Can you work these out from the model? Positions are in its coordinate system, mm. Face numbers are marked on the shaded views. A direction names the side the tool comes from. Coordinates: 2 decimals unless noted, no trailing zeros. Order: outer loops, then holes, each group sorted by start corner. A loop starts at its lowest first (then second) coordinate and runs counter-clockwise, first axis right, second up. Notation, with made-up numbers: (-30, -19) -> (12, -19) arc R21 ccw to (12, 14) -> close; hole circle Ø11 at (22.5, -13.5). An arc over 180 degrees is marked (long way). Write item = value, one per line. Start each with the question number.
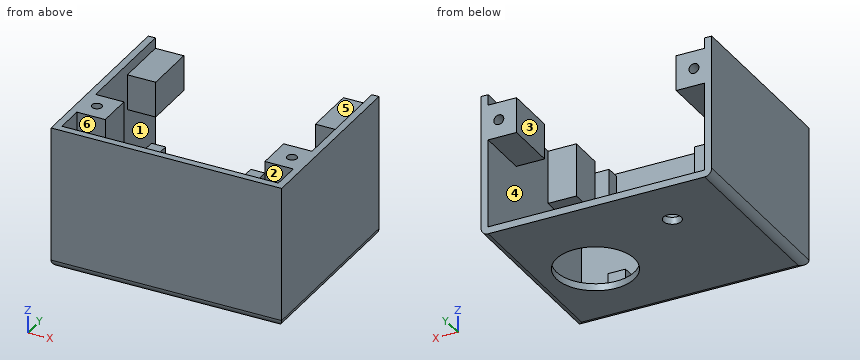
from build123d import *

# Parameters (mm, degrees)
SKETCH1_W           = 65
SKETCH1_H           = 52
BOSS_EXTRUDE1_DEPTH = 40
SHELL1_T            = -2
SKETCH7_W           = 10
SKETCH7_H           = 10
BOSS_EXTRUDE3_DEPTH = 15
SKETCH8_R           = 1.4
CUT_EXTRUDE3_DEPTH  = 10
SKETCH10_W          = 10
SKETCH10_H          = 10
BOSS_EXTRUDE4_DEPTH = 15
SKETCH11_R          = 1.4
CUT_EXTRUDE4_DEPTH  = 10
SKETCH13_R          = 2.5
CUT_EXTRUDE5_DEPTH  = 2
SKETCH16_W          = 10
SKETCH16_H          = 4
BOSS_EXTRUDE5_DEPTH = 13
SKETCH17_W          = 10
SKETCH17_H          = 2
CUT_EXTRUDE6_DEPTH  = 3
SKETCH18_W          = 4
SKETCH18_H          = 4
BOSS_EXTRUDE6_DEPTH = 10
SKETCH20_W          = 4
SKETCH20_H          = 4
BOSS_EXTRUDE7_DEPTH = 10
FILLET1_R           = 2
SKETCH22_W          = 5
SKETCH22_H          = 5
BOSS_EXTRUDE8_DEPTH = 3
SKETCH23_W          = 5
SKETCH23_H          = 5
BOSS_EXTRUDE9_DEPTH = 3
SKETCH24_R          = 11
CUT_EXTRUDE7_DEPTH  = 2


with BuildPart() as part:
    # Sketch1 → Boss-Extrude1 (new body)
    with BuildSketch(Plane.XY):
        with Locations((32.5, 26)):
            Rectangle(SKETCH1_W, SKETCH1_H)
    extrude(amount=BOSS_EXTRUDE1_DEPTH)

    # Shell1
    shell1_openings = [part.faces().sort_by_distance(p)[0] for p in [
        (32.5, 26, 40),
        (32.5, 52, 20),
    ]]
    offset(amount=SHELL1_T, openings=shell1_openings, kind=Kind.INTERSECTION)

    # Sketch7 → Boss-Extrude3 (add)
    with BuildSketch(Plane(origin=(0, 52, 0), x_dir=(1, 0, 0), z_dir=(0, 1, 0))):
        with Locations((5, -32)):
            Rectangle(SKETCH7_W, SKETCH7_H)
    boss_extrude3 = extrude(amount=-BOSS_EXTRUDE3_DEPTH)

    # Sketch8 → Cut-Extrude3 (cut)
    with BuildSketch(Plane(origin=(0, 52, 0), x_dir=(1, 0, 0), z_dir=(0, 1, 0))):
        with Locations((5, -32)):
            Circle(SKETCH8_R)
    cut_extrude3 = extrude(amount=-CUT_EXTRUDE3_DEPTH, mode=Mode.SUBTRACT)

    # Mirror3: Boss-Extrude3, Cut-Extrude3 across plane
    add(boss_extrude3.mirror(Plane(origin=(32.5, 0, 0), x_dir=(0, 0, 1), z_dir=(1, 0, 0))))
    add(cut_extrude3.mirror(Plane(origin=(32.5, 0, 0), x_dir=(0, 0, 1), z_dir=(1, 0, 0))), mode=Mode.SUBTRACT)

    # Sketch10 → Boss-Extrude4 (add)
    with BuildSketch(Plane.XY.offset(40)):
        with Locations((5, 15)):
            Rectangle(SKETCH10_W, SKETCH10_H)
    boss_extrude4 = extrude(amount=-BOSS_EXTRUDE4_DEPTH)

    # Sketch11 → Cut-Extrude4 (cut)
    with BuildSketch(Plane.XY.offset(40)):
        with Locations((5, 15)):
            Circle(SKETCH11_R)
    cut_extrude4 = extrude(amount=-CUT_EXTRUDE4_DEPTH, mode=Mode.SUBTRACT)

    # Mirror4: Boss-Extrude4, Cut-Extrude4 across plane
    add(boss_extrude4.mirror(Plane(origin=(32.5, 0, 0), x_dir=(0, 0, 1), z_dir=(1, 0, 0))))
    add(cut_extrude4.mirror(Plane(origin=(32.5, 0, 0), x_dir=(0, 0, 1), z_dir=(1, 0, 0))), mode=Mode.SUBTRACT)

    # Sketch13 → Cut-Extrude5 (cut)
    with BuildSketch(Plane(origin=(0, 0, 0), x_dir=(-1, 0, 0), z_dir=(0, 0, -1))):
        with Locations((-19, 37)):
            Circle(SKETCH13_R)
    extrude(amount=-CUT_EXTRUDE5_DEPTH, mode=Mode.SUBTRACT)

    # Sketch16 → Boss-Extrude5 (add)
    with BuildSketch(Plane.XY.offset(2)):
        with Locations((19, 6)):
            Rectangle(SKETCH16_W, SKETCH16_H)
    extrude(amount=BOSS_EXTRUDE5_DEPTH)

    # Sketch17 → Cut-Extrude6 (cut)
    with BuildSketch(Plane.XY.offset(15)):
        with Locations((19, 7)):
            Rectangle(SKETCH17_W, SKETCH17_H)
    extrude(amount=-CUT_EXTRUDE6_DEPTH, mode=Mode.SUBTRACT)

    # Sketch18 → Boss-Extrude6 (add)
    with BuildSketch(Plane.XY.offset(2)):
        with Locations((33, 46)):
            Rectangle(SKETCH18_W, SKETCH18_H)
    extrude(amount=BOSS_EXTRUDE6_DEPTH)

    # Sketch20 → Boss-Extrude7 (add)
    with BuildSketch(Plane.XY.offset(2)):
        with Locations((5, 46)):
            Rectangle(SKETCH20_W, SKETCH20_H)
    extrude(amount=BOSS_EXTRUDE7_DEPTH)

    # Fillet1
    fillet1_edges = [part.edges().sort_by_distance(p)[0] for p in [
        (65, 26, 0),
        (32.5, 0, 0),
        (0, 26, 0),
    ]]
    fillet(fillet1_edges, radius=FILLET1_R)

    # Sketch22 → Boss-Extrude8 (add)
    with BuildSketch(Plane.XY.offset(2)):
        with Locations((47.5, 37.8)):
            Rectangle(SKETCH22_W, SKETCH22_H)
    extrude(amount=BOSS_EXTRUDE8_DEPTH)

    # Sketch23 → Boss-Extrude9 (add)
    with BuildSketch(Plane.XY.offset(2)):
        with Locations((47.5, 10.2)):
            Rectangle(SKETCH23_W, SKETCH23_H)
    extrude(amount=BOSS_EXTRUDE9_DEPTH)

    # Sketch24 → Cut-Extrude7 (cut)
    with BuildSketch(Plane.XY.offset(2)):
        with Locations((47.5, 24.03)):
            Circle(SKETCH24_R)
    extrude(amount=-CUT_EXTRUDE7_DEPTH, mode=Mode.SUBTRACT)


solid = part.part
(1) If I drill on L1, parallel to Z at x = 60, y = 44.5; L2, parallel to Y at x = 56, z = 35; L3, parallel to X at y = 34, z = 19.5, over which ranges is the centre line in solid material (lowest first)? Write a range as from..to.
(2) For the marked faces 1, 2 and 3, which set-ups out of +Z, -Z, +X, -X, +Y, -Y let a thin tool reach every point of the face, with its end or its side?
(3) Thinking about a two-plate mould opening in Z: for the marked faces 4, 5 and 6, which applies, +Z half, -Z half, draft (parallel to the pull), parting line (faces both ways), or undercut?
(4) For P1, Ø6, axis at x = 32.5, y = 35.5, coming from the -Z side; P2, Ø1.5, axis at x = 48, y = 11, coming from the +Z side; P3, Ø2, axis at x = 5, z = 7, coming from the +Y side; P4, Ø0.6, axis at x = 21, y = 4.5, coming from the +Z side, each with a flat end and sliding along its axis, tell me the tip position at first contact or that it passes through.
(5) Imagine slicing it at C-C (z = 35). Write out the boundary of the cut face in (x, y).
(6) Imagine slicing it at D-D (x = 19). Write out the boundary of the cut face in (y, z).
(7) Imagine slicing it at A-A (y = 24.03). Write out the boundary of the cut face in (x, z).
(8) Imagine slicing it at B-B (x = 5). Write out the boundary of the cut face in (y, z), plus the area to 3 significant figures.
Result set:
q1.L1 = 0..2, 27..30.6, 33.4..37
q1.L2 = 0..2, 10..20, 37..52
q1.L3 = 0..2, 63..65
q2.face_1 = none
q2.face_2 = +Z
q2.face_3 = +Z, +Y
q3.face_4 = undercut
q3.face_5 = +Z half
q3.face_6 = draft
q4.P1 = 0
q4.P2 = 5
q4.P3 = 48
q4.P4 = 15
q5.outline = (0, 0) -> (65, 0) -> (65, 52) -> (55, 52) -> (55, 37) -> (63, 37) -> (63, 20) -> (55, 20) -> (55, 10) -> (63, 10) -> (63, 2) -> (2, 2) -> (2, 10) -> (10, 10) -> (10, 20) -> (2, 20) -> (2, 37) -> (10, 37) -> (10, 52) -> (0, 52) -> close; hole circle Ø2.8 at (5, 15); hole circle Ø2.8 at (60, 15)
q6.outline = (0, 2) arc R2 ccw to (2, 0) -> (34.5, 0) -> (34.5, 2) -> (8, 2) -> (8, 12) -> (6, 12) -> (6, 15) -> (4, 15) -> (4, 2) -> (2, 2) -> (2, 40) -> (0, 40) -> close; (39.5, 0) -> (52, 0) -> (52, 2) -> (39.5, 2) -> close
q7.outline = (0, 2) arc R2 ccw to (2, 0) -> (36.5, 0) -> (36.5, 2) -> (2, 2) -> (2, 40) -> (0, 40) -> close; (58.5, 0) -> (63, 0) arc R2 ccw to (65, 2) -> (65, 40) -> (63, 40) -> (63, 2) -> (58.5, 2) -> close
q8.outline = (0, 2) arc R2 ccw to (2, 0) -> (52, 0) -> (52, 2) -> (48, 2) -> (48, 12) -> (44, 12) -> (44, 2) -> (2, 2) -> (2, 40) -> (0, 40) -> close; (10, 25) -> (20, 25) -> (20, 40) -> (16.4, 40) -> (16.4, 30) -> (13.6, 30) -> (13.6, 40) -> (10, 40) -> close; (37, 27) -> (52, 27) -> (52, 30.6) -> (42, 30.6) -> (42, 33.4) -> (52, 33.4) -> (52, 37) -> (37, 37) -> close
q8.area = 463 mm2
